```python
from build123d import *

# Parameters (mm, degrees)
R_VOLUTION1_ANGLE       = 45
ENL_V_MAT_EXTRU_1_DEPTH = 25
ENL_V_MAT_EXTRU_2_DEPTH = 64
ENL_V_MAT_EXTRU_3_DEPTH = 64


with BuildPart() as part:
    # Esquisse1 → Révolution1 (revolve, symmetric)
    with BuildSketch(Plane.XY) as r_volution1_sk:
        Polygon((-127, 31.5), (-97, 31.5), (-97, 28.5), (-100, 28.5), (-100, 25.5), (-97, 25.5), (-97, 22.5), (-100, 22.5), (-100, -22.5), (-97, -22.5), (-97, -25.5), (-100, -25.5), (-100, -28.5), (-97, -28.5), (-97, -31.5), (-127, -31.5), align=None)
    revolve(axis=Axis((0, 55, 0), (0, -1, 0)), revolution_arc=R_VOLUTION1_ANGLE / 2)
    revolve(r_volution1_sk.sketch, axis=Axis((0, 55, 0), (0, 1, 0)), revolution_arc=R_VOLUTION1_ANGLE / 2)

    # Esquisse3 → Enlèv. mat.-Extru.1 (cut, symmetric)
    with BuildSketch(Plane(origin=(0, 0, 0), x_dir=(1, 0, 0), z_dir=(0, 1, 0))):
        Polygon((-127, 50.133100711), (-90.465463023, 35), (-90.465463023, -35), (-127, 0.133100711), align=None)
    extrude(amount=ENL_V_MAT_EXTRU_1_DEPTH, both=True, mode=Mode.SUBTRACT)

    # Esquisse4 → Enlèv. mat.-Extru.2 (cut, through all)
    with BuildSketch(Plane(origin=(0, 31.5, 0), x_dir=(1, 0, 0), z_dir=(0, 1, 0))):
        with BuildLine():
            Line((-117.332700629, -48.60079591), (-89.616314654, -37.120292939))
            Line((-89.616314654, -37.120292939), (-126.704281868, -8.661694766))
            ThreePointArc((-126.704281868, -8.661694766), (-123.641801817, -29.012149926), (-117.332700629, -48.60079591))
        make_face()
    extrude(amount=-ENL_V_MAT_EXTRU_2_DEPTH, mode=Mode.SUBTRACT)

    # Esquisse5 → Enlèv. mat.-Extru.3 (cut, through all)
    with BuildSketch(Plane(origin=(0, 31.5, 0), x_dir=(1, 0, 0), z_dir=(0, 1, 0))):
        Polygon((-126.704281868, -8.661694766), (-148.461378706, 8.033112817), (-117.332700629, 48.60079591), (-103.474507641, 42.860544425), align=None)
    extrude(amount=-ENL_V_MAT_EXTRU_3_DEPTH, mode=Mode.SUBTRACT)


solid = part.part
```
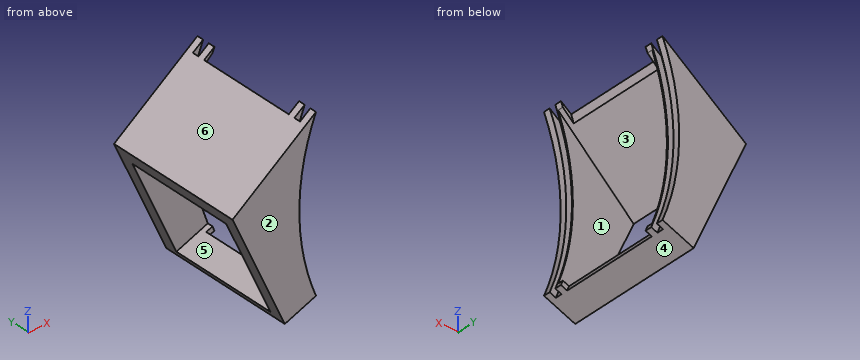
For this review, take the finished solid that the model builds, in its own axes (mm). Face numbers are marked on the shaded views. A direction names the side the tool comes from. Round coordinates to 2 decimals unless told otherwise and drop trailing zeros. Order: outer loops, then holes, each group sorted by start corner. A loop starts at its lowest first (then second) coordinate and runs counter-clockwise, first axis right, second up.
Q1. We need section A-A, the plane y = -4.5. Give the boundary of the cut face in (x, z).
Findings below:
outline: (-126.7, 8.66) - (-124.03, 2.73) - (-95.28, 30.37) arc R100 cw to (-94.18, 33.62) - close; (-104.41, -40.78) - (-103.47, -42.86) - (-92.39, -38.27) arc R100 cw to (-93.24, -36.15) - close
Q2. We need section D-D, the plane y = 23.5. Give the boundary of the cut face in (x, z), plus the area to 3 significant figures.
Findings below:
outline: (-126.7, 8.66) - (-124.03, 2.73) - (-90.47, 35) arc R97 cw to (-89.62, 37.12) - close; (-104.41, -40.78) - (-103.47, -42.86) - (-89.62, -37.12) arc R97 cw to (-90.47, -35) - close
area: 204 mm2
Q3. Insertion check: P1, Ø5, axis at x = -94, z = 1, coming from the +Y side; P2, Ø1, axis at x = -115, y = -7, coming from the -Z side; P3, Ø8.5, axis at x = -92.5, z = -13, coming from the +Y side. Each pin has a flat end and moves straight along its axis. Give the tip position at first contact, or say it passes through.
Findings below:
P1: passes through
P2: stops at z = 10.93
P3: stops at y = 31.5
Q4. Mouldability with a two-part tool opening along Y and no side actions: class the marked faces 1, 2, 3 and 4 as pulls with the +Y half, pulls with the -Y half, needs draft (parallel to the pull), parting line crosses it, or undercut.
Findings below:
face 1: undercut
face 2: pulls with the -Y half
face 3: undercut
face 4: needs draft
Q5. We need section C-C, the plane x = -107. Give the boundary of the cut face in (y, z).
Findings below:
outline: (-31.5, -35.04) - (-25, -35.04) - (-25, 19.1) - (25, 19.1) - (25, -35.04) - (31.5, -35.04) - (31.5, 23.78) - (-31.5, 23.78) - close
Q6. We need section B-B, the plane z = -4. Give the boundary of the cut face in (x, y).
Findings below:
outline: (-121, -31.5) - (-96.92, -31.5) - (-96.92, -28.5) - (-99.92, -28.5) - (-99.92, -25.5) - (-96.92, -25.5) - (-96.92, -25) - (-121, -25) - close; (-121, 25) - (-96.92, 25) - (-96.92, 25.5) - (-99.92, 25.5) - (-99.92, 28.5) - (-96.92, 28.5) - (-96.92, 31.5) - (-121, 31.5) - close
Q7. Machinability: for the marked faces 5 and 6, which of the approach directions +Z, -Z, +X, -X, +Y, -Y give a long, thin tool a straight path to every point of the face, cutting with its end or side? Answer none if there is none.
Findings below:
face 5: -X
face 6: +Z, -X, +Y, -Y
Q8. Wall thickness on line 1 (Y direction, x = -98, z = -16.5); line 2 (Y direction, x = -105, z = -34.5); line 3 (Z direction, x = -103, y = -8): over which ranges is each line inside the solid? List them lowest first.
Findings below:
line 1: y = -31.5 to -28.5, -25.5 to -25, 25 to 25.5, 28.5 to 31.5
line 2: y = -31.5 to -25, 25 to 31.5
line 3: z = -42.66 to -40.19, 22.95 to 26.85
